```python
from build123d import *

# Parameters (mm, degrees)
SKETCH1_R           = 48.26
BOSS_EXTRUDE1_DEPTH = 38.1
SKETCH2_R           = 21.59
BOSS_EXTRUDE2_DEPTH = 33.02
SKETCH3_W           = 19.05
SKETCH3_H           = 22.86
BOSS_EXTRUDE3_DEPTH = 56.388


with BuildPart() as part:
    # Sketch1 → Boss-Extrude1 (new body)
    with BuildSketch(Plane.XY):
        with Locations(Location((0, 0, 0), (0, 0, 180))):
            Circle(SKETCH1_R)
    extrude(amount=BOSS_EXTRUDE1_DEPTH)

    # Sketch2 → Boss-Extrude2 (add)
    with BuildSketch(Plane(origin=(0, 0, 0), x_dir=(-1, 0, 0), z_dir=(0, 0, -1))):
        Circle(SKETCH2_R)
    extrude(amount=BOSS_EXTRUDE2_DEPTH)

    # Sketch3 → Boss-Extrude3 (add)
    with BuildSketch(Plane(origin=(0, 0, 0), x_dir=(1, 0, 0), z_dir=(0, 1, 0))):
        with Locations((0, -19.05)):
            Rectangle(SKETCH3_W, SKETCH3_H)
    extrude(amount=-BOSS_EXTRUDE3_DEPTH)


solid = part.part
```
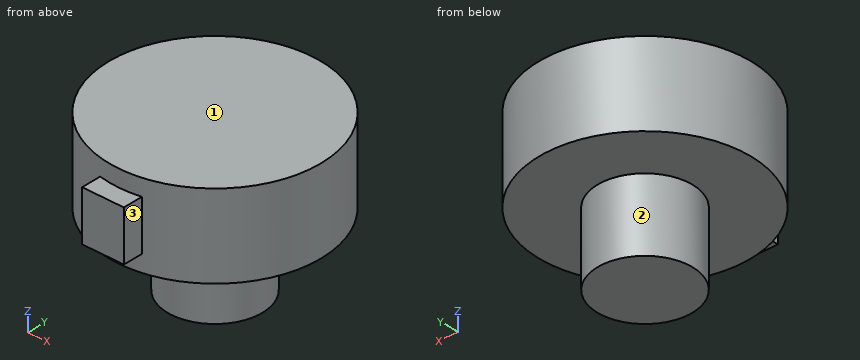
Part model, mm, in its own coordinate system. Face numbers are marked on the shaded views. A direction names the side the tool comes from. Round coordinates to 2 decimals unless told otherwise and drop trailing zeros. Loops run counter-clockwise (first coordinate to the right, second up) from the corner with the lowest first, then second, coordinate; pieces in that order, holes last.
Item 1: Drop flat-ended pins along their axis: P1, Ø3, axis at x = -22.5, y = 26.5, coming from the -Z side; P2, Ø7.5, axis at y = -54, z = 19, coming from the -X side (3 decimals); P3, Ø8, axis at y = -13.5, z = -22, coming from the -X side. Give the stop position or say it passes through.
Item 2: Cut at B-B, the plane x = 0. Give the cut face in (y, z), then the cut area to 3 significant figures.
Item 3: Cut at D-D, the plane y = -15.5. Give the cut face in (x, z).
Item 4: Cut at A-A, the plane y = 0. Give the cut face in (x, z).
Item 5: 3-axis set-ups, long thin cutter, end or side, ignore diameter. For the marked faces 1, 2 and 3: which of +Z, -Z, +X, -X, +Y, -Y reach the whole face in a straight line?
Item 6: Cut at C-C, the plane z = 17.5. Give the cut face in (x, y) (3 decimals), then the cut area to 3 significant figures.
Item 7: Drill centre lines: line 1 (Z direction, x = -30.5, y = 35.5); line 2 (X direction, y = 1, z = -25); line 3 (Y direction, x = 22, z = 17). Where is each one in solid material? Low to high.
A:
1. P1: stops at z = 0
1. P2: stops at x = -9.525
1. P3: stops at x = -19.39
2. outline: (-56.39, 7.62) - (-48.26, 7.62) - (-48.26, 0) - (-21.59, 0) - (-21.59, -33.02) - (21.59, -33.02) - (21.59, 0) - (48.26, 0) - (48.26, 38.1) - (-48.26, 38.1) - (-48.26, 30.48) - (-56.39, 30.48) - close
2. area: 5,290 mm2
3. outline: (-45.7, 0) - (-15.03, 0) - (-15.03, -33.02) - (15.03, -33.02) - (15.03, 0) - (45.7, 0) - (45.7, 38.1) - (-45.7, 38.1) - close
4. outline: (-48.26, 0) - (-21.59, 0) - (-21.59, -33.02) - (21.59, -33.02) - (21.59, 0) - (48.26, 0) - (48.26, 38.1) - (-48.26, 38.1) - close
5. face 1: +Z, +X, -X, +Y, -Y
5. face 2: -Z
5. face 3: +Z, -Z, +X, -Y
6. outline: (-9.525, -56.388) - (9.525, -56.388) - (9.525, -47.311) arc R48.26 ccw (long way) to (-9.525, -47.311) - close
6. area: 7,480 mm2
7. line 1: z = 0 to 38.1
7. line 2: x = -21.57 to 21.57
7. line 3: y = -42.95 to 42.95
